Here's how the part is built. I have some questions about the finished solid (model axes, mm). Face numbers are marked on the shaded views. A direction names the side the tool comes from. Coordinates: 2 decimals unless noted, no trailing zeros. Loops run counter-clockwise (first coordinate to the right, second up) from the corner with the lowest first, then second, coordinate; pieces in that order, holes last. Notation, with made-up numbers: M 47.25,16 L 92.25,16 A19 cw 92.25,38 Z; hole C 13,34.5 d7. An arc over 180 degrees is marked long. Use one line per item in the form item = value. Start each with the question number.
(1) Imagine slicing it at D-D, the plane x = 1. Please give me the cut outline in (y, z), and give its area (3 significant figures).
(2) Imagine slicing it at C-C, the plane y = -4. Please give me the cut outline in (x, z).
(3) Imagine slicing it at B-B, the plane z = -18.5. Please give me the cut outline in (x, y).
(4) Please list where these lines run through material, in increasing order: L1, parallel to X at y = -2.25, z = -16.5; L2, parallel to X at y = -0.5, z = 16; L3, parallel to Z at x = 27.5, y = -5.
(5) Will these pins go through, and if not, where does the flat tip stop? P1, Ø1.4, axis at y = -1, z = 19.5, coming from the +X side; P2, Ø2, axis at x = -1, y = -4, coming from the +Z side; P3, Ø5, axis at x = 18, z = 17.5, coming from the +Y side; P4, Ø5.5, axis at x = 22, z = -2.5, coming from the -Y side.
(6) Imagine slicing it at A-A, the plane x = 20.5. Please give me the cut outline in (y, z).
(7) Thinking about a two-plate mould opening in Z: for the marked faces 1, 2, 3 and 4, which applies, +Z half, -Z half, draft (parallel to the pull), parting line (faces both ways), or undercut?
(8) On a 3-axis mill with a long thin cutter (end or side, diameter ignored), from which of +Z, -Z, +X, -X, +Y, -Y can I reach the whole of each face in a straight line? I mean the marked faces 5, 6 and 7. Say none if no direction works.
```python
from build123d import *

# Parameters (mm, degrees)
F1_DEPTH = 8
F2_DEPTH = 1.3
F3_DEPTH = 2.6
F4_DEPTH = 1.3
F5_DEPTH = 1.2
F6_R     = 5
F7_R     = 0.5


with BuildPart() as f1:
    # F0 (on Front) → F1 (new body)
    with BuildSketch(Plane.XZ):
        with BuildLine():
            Line((6, -22.5), (30, -22.5))
            Line((30, -22.5), (30, -5.5))
            Line((30, -5.5), (21.4, -5.5))
            ThreePointArc((21.4, -5.5), (17.5109127035, -3.8890872965), (15.9, 0))
            ThreePointArc((15.9, 0), (17.5109127035, 3.8890872965), (21.4, 5.5))
            Line((21.4, 5.5), (30, 5.5))
            Line((30, 5.5), (30, 22.5))
            Line((30, 22.5), (4.2, 22.5))
            Line((4.2, 22.5), (4.2, 15.5500004172))
            ThreePointArc((4.2, 15.5500004172), (2.969848481, 12.5801519362), (0, 11.3500004172))
            ThreePointArc((0, 11.3500004172), (-2.969848481, 12.5801519362), (-4.2, 15.5500004172))
            Line((-4.2, 15.5500004172), (-4.2, 22.5))
            Line((-4.2, 22.5), (-30, 22.5))
            Line((-30, 22.5), (-30, 4.2))
            Line((-30, 4.2), (-23.05, 4.2))
            ThreePointArc((-23.05, 4.2), (-20.080151519, 2.969848481), (-18.85, 0))
            ThreePointArc((-18.85, 0), (-20.080151519, -2.969848481), (-23.05, -4.2))
            Line((-23.05, -4.2), (-30, -4.2))
            Line((-30, -4.2), (-30, -22.5))
            Line((-30, -22.5), (-6, -22.5))
            Line((-6, -22.5), (-6, -16.5))
            ThreePointArc((-6, -16.5), (-4.2426406871, -12.2573593129), (0, -10.5))
            ThreePointArc((0, -10.5), (4.2426406871, -12.2573593129), (6, -16.5))
            Line((6, -16.5), (6, -22.5))
        make_face()
    extrude(amount=F1_DEPTH)

    # F0 (on Front) → F2 (join)
    with BuildSketch(Plane.XZ):
        with BuildLine():
            Line((-30, -3.05), (-30, -4.2))
            Line((-30, -4.2), (-23.05, -4.2))
            ThreePointArc((-23.05, -4.2), (-20.080151519, -2.969848481), (-18.85, 0))
            ThreePointArc((-18.85, 0), (-20.080151519, 2.969848481), (-23.05, 4.2))
            Line((-23.05, 4.2), (-30, 4.2))
            Line((-30, 4.2), (-30, 3.05))
            Line((-30, 3.05), (-23.05, 3.05))
            ThreePointArc((-23.05, 3.05), (-20.8933243174, 2.1566756826), (-20, 0))
            ThreePointArc((-20, 0), (-20.8933243174, -2.1566756826), (-23.05, -3.05))
            Line((-23.05, -3.05), (-30, -3.05))
        make_face()
    extrude(amount=F2_DEPTH)

    # F0 (on Front) → F3 (join)
    with BuildSketch(Plane.XZ):
        with BuildLine():
            Line((21.4, -5.5), (30, -5.5))
            Line((30, -5.5), (30, -3.7))
            Line((30, -3.7), (21.4, -3.7))
            ThreePointArc((21.4, -3.7), (18.7837049096, -2.6162950904), (17.7, 0))
            ThreePointArc((17.7, 0), (18.7837049096, 2.6162950904), (21.4, 3.7))
            Line((21.4, 3.7), (30, 3.7))
            Line((30, 3.7), (30, 5.5))
            Line((30, 5.5), (21.4, 5.5))
            ThreePointArc((21.4, 5.5), (17.5109127035, 3.8890872965), (15.9, 0))
            ThreePointArc((15.9, 0), (17.5109127035, -3.8890872965), (21.4, -5.5))
        make_face()
    extrude(amount=F3_DEPTH)

    # F0 (on Front) → F4 (join)
    with BuildSketch(Plane.XZ):
        with BuildLine():
            Line((4.2, 15.5500004172), (4.2, 22.5))
            Line((4.2, 22.5), (3.05, 22.5))
            Line((3.05, 22.5), (3.05, 15.5500004172))
            ThreePointArc((3.05, 15.5500004172), (2.1566756826, 13.3933247346), (0, 12.5000004172))
            ThreePointArc((0, 12.5000004172), (-2.1566756826, 13.3933247346), (-3.05, 15.5500004172))
            Line((-3.05, 15.5500004172), (-3.05, 22.5))
            Line((-3.05, 22.5), (-4.2, 22.5))
            Line((-4.2, 22.5), (-4.2, 15.5500004172))
            ThreePointArc((-4.2, 15.5500004172), (-2.969848481, 12.5801519362), (0, 11.3500004172))
            ThreePointArc((0, 11.3500004172), (2.969848481, 12.5801519362), (4.2, 15.5500004172))
        make_face()
    extrude(amount=F4_DEPTH)

    # F0 (on Front) → F5 (join)
    with BuildSketch(Plane.XZ):
        with BuildLine():
            Line((4, -22.5), (6, -22.5))
            Line((6, -22.5), (6, -16.5))
            ThreePointArc((6, -16.5), (4.2426406871, -12.2573593129), (0, -10.5))
            ThreePointArc((0, -10.5), (-4.2426406871, -12.2573593129), (-6, -16.5))
            Line((-6, -16.5), (-6, -22.5))
            Line((-6, -22.5), (-4, -22.5))
            Line((-4, -22.5), (-4, -16.5))
            ThreePointArc((-4, -16.5), (-2.8284271247, -13.6715728753), (0, -12.5))
            ThreePointArc((0, -12.5), (2.8284271247, -13.6715728753), (4, -16.5))
            Line((4, -16.5), (4, -22.5))
        make_face()
    extrude(amount=F5_DEPTH)

    # F6
    f6_edges = [f1.edges().sort_by_distance(p)[0] for p in [
        (-30, -4, 22.5),
        (30, -4, 22.5),
        (-30, -4, -22.5),
        (30, -4, -22.5),
    ]]
    fillet(f6_edges, radius=F6_R)

    # F7
    f7_edges = [f1.edges().sort_by_distance(p)[0] for p in [
        (-30, -0.65, 3.05),
        (-30, -0.65, -3.05),
        (30, -1.3, 3.7),
        (30, -1.3, -3.7),
        (4, -0.6, -22.5),
        (-4, -0.6, -22.5),
        (3.05, -0.65, 22.5),
        (-3.05, -0.65, 22.5),
    ]]
    fillet(f7_edges, radius=F7_R)


solid = f1.part
```
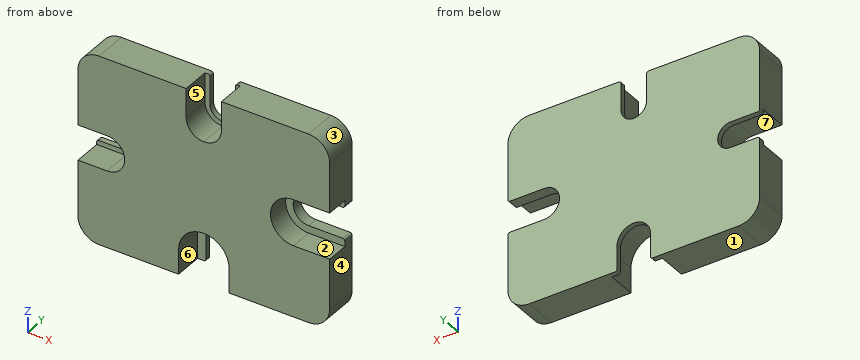
Answer:
q1.outline = M -8,-10.58 L -1.2,-10.58 L -1.2,-12.63 L 0,-12.63 L 0,12.67 L -1.3,12.67 L -1.3,11.47 L -8,11.47 Z
q1.area = 180 mm²
q2.outline = M -30,-17.5 A5 ccw -25,-22.5 L -6,-22.5 L -6,-16.5 A6 cw 6,-16.5 L 6,-22.5 L 25,-22.5 A5 ccw 30,-17.5 L 30,-5.5 L 21.4,-5.5 A5.5 cw 21.4,5.5 L 30,5.5 L 30,17.5 A5 ccw 25,22.5 L 4.2,22.5 L 4.2,15.55 A4.2 cw -4.2,15.55 L -4.2,22.5 L -25,22.5 A5 ccw -30,17.5 L -30,4.2 L -23.05,4.2 A4.2 cw -23.05,-4.2 L -30,-4.2 Z
q3.outline = M -29.9,-8 L -6,-8 L -6,-1.2 L -4,-1.2 L -4,0 L -29.9,0 Z; M 4,-1.2 L 6,-1.2 L 6,-8 L 29.9,-8 L 29.9,0 L 4,0 Z
q4.L1 = -30 to -6, 6 to 30
q4.L2 = -30 to -3.05, 3.05 to 30
q4.L3 = -21.83 to -5.5, 5.5 to 21.83
q5.P1 = 29.83
q5.P2 = 11.86
q5.P3 = 0
q5.P4 = -2.6
q6.outline = M -8,-22.5 L 0,-22.5 L 0,-3.59 L -2.6,-3.59 L -2.6,-5.43 L -8,-5.43 Z; M -8,5.43 L -2.6,5.43 L -2.6,3.59 L 0,3.59 L 0,22.5 L -8,22.5 Z
q7.face_1 = -Z half
q7.face_2 = undercut
q7.face_3 = +Z half
q7.face_4 = draft
q8.face_5 = +Z, -Y
q8.face_6 = -Z, -Y
q8.face_7 = -X, -Y
